from build123d import *

# Parameters (mm, degrees)
SKETCH1_W           = 9.97
SKETCH1_H           = 2.17
BOSS_EXTRUDE1_DEPTH = 4.07
SKETCH1_3_W         = 1.75
SKETCH1_3_H         = 0.63
BOSS_EXTRUDE2_DEPTH = 0.2


with BuildPart() as part:
    # Sketch1 → Boss-Extrude1 (new body)
    with BuildSketch(Plane.XY):
        with Locations((0, 2.505440613)):
            Rectangle(SKETCH1_W, SKETCH1_H)
    extrude(amount=BOSS_EXTRUDE1_DEPTH)

    # Sketch1_3 → Boss-Extrude2 (add)
    with BuildSketch(Plane.XY):
        with Locations((0, 1.105440613)):
            Rectangle(SKETCH1_3_W, SKETCH1_3_H)
    extrude(amount=BOSS_EXTRUDE2_DEPTH)

    # Sketch2 → Revolve1 (revolve)
    with BuildSketch(Plane.XY.offset(1.78)):
        with BuildLine():
            Line((-3.005, 1.420440613), (-4.605, 1.420440613))
            Line((-4.605, 1.420440613), (-4.605, 1.380440613))
            ThreePointArc((-4.605, 1.380440613), (-4.13637085, 0.249069763), (-3.005, -0.219559387))
            Line((-3.005, -0.219559387), (-3.005, 1.420440613))
        make_face()
    revolve(axis=Axis((-3.005, 1.420440613, 1.78), (0, -1, 0)))

    # Sketch3 one side → Revolve2 (revolve)
    with BuildSketch(Plane.XY.offset(1.9)):
        with BuildLine():
            ThreePointArc((3.105, 0.020440613), (4.23637085, 0.489069763), (4.705, 1.620440613))
            Line((4.705, 1.620440613), (3.105, 1.620440613))
            Line((3.105, 1.620440613), (3.105, 0.020440613))
        make_face()
    revolve(axis=Axis((3.105, 1.620440613, 1.9), (0, -1, 0)))


solid = part.part
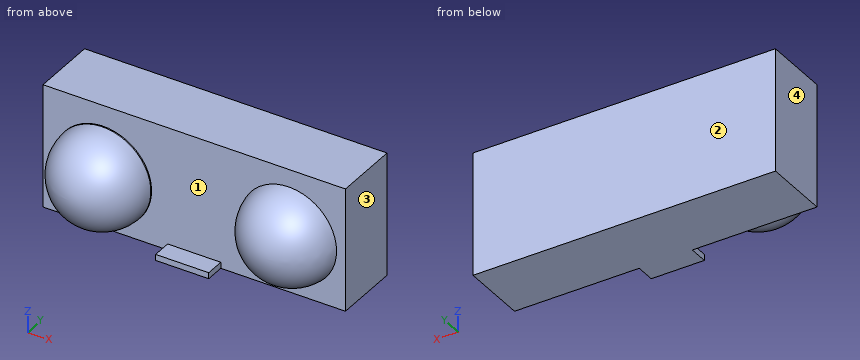
Build history of the part. All positions in model axes, mm. Face numbers are marked on the shaded views. Coordinates: 2 decimals unless noted, no trailing zeros. Order: outer loops, then holes, each group sorted by start corner. A loop starts at its lowest first (then second) coordinate and runs counter-clockwise, first axis right, second up. Notation, with made-up numbers: (58.25, 8.25) - (92.25, 8.25) arc R21 ccw to (92.25, 43.25) - close; hole circle Ø7 at (23.5, -25). An arc over 180 degrees is marked (long way). Write each question's results on one line, items separated by ' | '. Start each with the question number.
Item 1: Mould opens along X. For the marked faces 1, 2, 3 and 4 say: released by +X, released by -X, zero draft, split by the parting line, or undercut.
Item 2: Band-saw the part on A-A on z = 1.45. Write the cut outline in (x, y) (3 decimals).
Item 3: Band-saw the part on B-B on x = 0. Write the cut outline in (y, z).
Item 4: Band-saw the part on C-C on z = 2.3. Write the cut outline in (x, y) (3 decimals).
Item 5: Band-saw the part on D-D on x = -3.5. Write the cut outline in (y, z).
Item 6: Wall check: probe 1 along Y at (x, z) = (-2.25, 1.5); probe 2 along Y at (x, z) = (1, 2.3); probe 3 along X at (y, z) = (0.6, 2.75). Give the ranges that are in metal, low to high. Write a range as [from, to].
Item 7: Flat gauge pins, fed straight in: pin 1 (1.5 mm diameter, centred on x = -0.5, z = 0.5, fed in from -Y); pin 2 (1.2 mm diameter, centred on x = -1.5, z = 2, fed in from -Y); pin 3 (0.5 mm diameter, centred on x = 0, y = 1, fed in from +Z). Where does each tip first touch, or does it go through?
Numbers:
1) face 1: undercut | face 2: zero draft | face 3: released by +X | face 4: released by -X
2) outline: (-4.985, 1.42) - (-4.571, 1.42) - (-4.571, 1.38) arc R1.566 ccw to (-1.439, 1.38) - (-1.439, 1.42) - (1.583, 1.42) arc R1.535 ccw to (4.627, 1.42) - (4.985, 1.42) - (4.985, 3.59) - (-4.985, 3.59) - close
3) outline: (0.79, 0) - (3.59, 0) - (3.59, 4.07) - (1.42, 4.07) - (1.42, 0.2) - (0.79, 0.2) - close
4) outline: (-4.985, 1.42) - (-4.518, 1.42) - (-4.518, 1.38) arc R1.513 ccw to (-1.492, 1.38) - (-1.492, 1.42) - (1.569, 1.42) arc R1.549 ccw to (4.641, 1.42) - (4.985, 1.42) - (4.985, 3.59) - (-4.985, 3.59) - close
5) outline: (1.38, 0.26) - (1.42, 0.26) - (1.42, 0) - (3.59, 0) - (3.59, 4.07) - (1.42, 4.07) - (1.42, 3.3) - (1.38, 3.3) arc R1.52 ccw to start
6) probe 1: [0, 3.59] | probe 2: [1.42, 3.59] | probe 3: [-4.01, -2], [2.21, 4]
7) pin 1: y = 0.79 | pin 2: y = 0.07 | pin 3: z = 0.2
